```python
from build123d import *

# Parameters (mm, degrees)
F0_W      = 1348.74
F0_H      = 685.8
F1_DEPTH  = 25.4
F3_W      = 50.8
F3_H      = 317.5
F4_DEPTH  = 38.1
F5_W      = 50.8
F5_H      = 76.2
F6_DEPTH  = 660.4
F8_DEPTH  = 25.4
F9_W      = 1194.675028
F9_H      = 25.596991
F10_DEPTH = 304.8
F11_R     = 25.4
F12_R     = 25.4
F13_R     = 25.4
F14_R     = 25.4


with BuildPart() as f1:
    # F0 (on Top) → F1 (new body)
    with BuildSketch(Plane.XY):
        Rectangle(F0_W, F0_H)
    extrude(amount=F1_DEPTH)

    # F3 (on face) → F4 (join)
    with BuildSketch(Plane.XY.offset(25.4)):
        with Locations((-623.57, 44.45)):
            Rectangle(F3_W, F3_H)
        with Locations((623.57, 44.45)):
            Rectangle(F3_W, F3_H)
    extrude(amount=F4_DEPTH)

    # F5 (on face) → F6 (join)
    with BuildSketch(Plane.XY.offset(25.4)):
        with Locations((-623.57, -152.4)):
            Rectangle(F5_W, F5_H)
        with Locations((623.57, -152.4)):
            Rectangle(F5_W, F5_H)
    extrude(amount=F6_DEPTH)

    # F7 (on face) → F8 (join)
    with BuildSketch(Plane.XY.offset(685.8)):
        with BuildLine():
            ThreePointArc((-623.57, 241.3), (-641.530512, 233.860512), (-648.97, 215.9))
            Line((-648.97, 215.9), (-648.97, -241.3))
            ThreePointArc((-648.97, -241.3), (-641.530512, -259.260512), (-623.57, -266.7))
            ThreePointArc((-623.57, -266.7), (-605.609488, -259.260512), (-598.17, -241.3))
            Line((-598.17, -241.3), (-598.17, 215.9))
            ThreePointArc((-598.17, 215.9), (-605.609488, 233.860512), (-623.57, 241.3))
        make_face()
        with BuildLine():
            Line((648.97, -241.3), (648.97, 215.9))
            ThreePointArc((648.97, 215.9), (641.530512, 233.860512), (623.57, 241.3))
            ThreePointArc((623.57, 241.3), (605.609488, 233.860512), (598.17, 215.9))
            Line((598.17, 215.9), (598.17, -241.3))
            ThreePointArc((598.17, -241.3), (605.609488, -259.260512), (623.57, -266.7))
            ThreePointArc((623.57, -266.7), (641.530512, -259.260512), (648.97, -241.3))
        make_face()
    extrude(amount=F8_DEPTH)

    # F9 (on face) → F10 (join)
    with BuildSketch(Plane.XY.offset(25.4)):
        with Locations((-0.20507, -145.966001)):
            Rectangle(F9_W, F9_H)
    extrude(amount=F10_DEPTH)

    # F11
    f11_edges = [f1.edges().sort_by_distance(p)[0] for p in [
        (-674.37, 342.9, 12.7),
    ]]
    fillet(f11_edges, radius=F11_R)

    # F12
    f12_edges = [f1.edges().sort_by_distance(p)[0] for p in [
        (-674.37, -342.9, 12.7),
    ]]
    fillet(f12_edges, radius=F12_R)

    # F13
    f13_edges = [f1.edges().sort_by_distance(p)[0] for p in [
        (674.37, -342.9, 12.7),
    ]]
    fillet(f13_edges, radius=F13_R)

    # F14
    f14_edges = [f1.edges().sort_by_distance(p)[0] for p in [
        (674.37, 342.9, 12.7),
    ]]
    fillet(f14_edges, radius=F14_R)


solid = f1.part
```
The model under review builds one solid part; all positions refer to its coordinate system, in mm. A direction names the side the tool comes from. Round coordinates to 2 decimals unless told otherwise and drop trailing zeros. Order: outer loops, then holes, each group sorted by start corner. A loop starts at its lowest first (then second) coordinate and runs counter-clockwise, first axis right, second up.
(1) Take a section at A-A, the plane y = 17. State the section outline as (x, z) points.
Working result:
outline: (-674.37, 0) - (674.37, 0) - (674.37, 25.4) - (648.97, 25.4) - (648.97, 63.5) - (598.17, 63.5) - (598.17, 25.4) - (-598.17, 25.4) - (-598.17, 63.5) - (-648.97, 63.5) - (-648.97, 25.4) - (-674.37, 25.4) - close; (-648.97, 685.8) - (-598.17, 685.8) - (-598.17, 711.2) - (-648.97, 711.2) - close; (598.17, 685.8) - (648.97, 685.8) - (648.97, 711.2) - (598.17, 711.2) - close
(2) Wall thickness on L1, parallel to Z at x = -406, y = -289.5; L2, parallel to Y at x = 490.5, z = 177.5; L3, parallel to Y at x = 602.5, z = 188.5: over which ranges is each line inside the solid? List them lowest first.
Working result:
L1: z = 0 to 25.4
L2: y = -158.76 to -133.17
L3: y = -190.5 to -114.3
(3) Mouldability with a two-part tool opening along X and no side actions: class faces 5 (the face through (666.73, -335.66, 12.88)), 6 (the face through (598.17, -115, 341)), 7 (the face through (623, -9, 711.2)) as released by +X, released by -X, zero draft, split by the parting line, or undercut.
Working result:
face 5: released by +X
face 6: undercut
face 7: zero draft
(4) Tool access review of faces 1 (the face through (623, 47, 63.5)), 2 (the face through (-9, -133.168, 176)), 3 (the face through (623, -228, 685.8)), 4 (the face through (648.97, -115, 341)): name each direction out of +Z, -Z, +X, -X, +Y, -Y from which nothing blocks a thin tool from reaching the whole face with its end or side.
Working result:
face 1: +X, -X, +Y
face 2: +Z, +Y
face 3: +X, -X, -Y
face 4: +Z, +X, +Y, -Y
(5) Take a section at B-B, the plane z = 257. State the section outline as (x, y) points, plus the area to 3 significant figures.
Working result:
outline: (-648.97, -190.5) - (-598.17, -190.5) - (-598.17, -114.3) - (-648.97, -114.3) - close; (-597.54, -158.76) - (597.13, -158.76) - (597.13, -133.17) - (-597.54, -133.17) - close; (598.17, -190.5) - (648.97, -190.5) - (648.97, -114.3) - (598.17, -114.3) - close
area: 38,300 mm2
(6) Take a section at D-D, the plane x = 148.5. State the section outline as (y, z) points, plus the area to 3 significant figures.
Working result:
outline: (-342.9, 0) - (342.9, 0) - (342.9, 25.4) - (-133.17, 25.4) - (-133.17, 330.2) - (-158.76, 330.2) - (-158.76, 25.4) - (-342.9, 25.4) - close
area: 25,200 mm2
(7) For P1, Ø1.5, axis at x = 272, z = 323.5, coming from the +Y side; P2, Ø6, axis at y = -174, z = 157.5, coming from the +X side; P3, Ø1, axis at x = 147, y = 47, coming from the +Z side, all flat-tipped, find the tip position at first contact; note any pin that passes through.
Working result:
P1: stops at y = -133.17
P2: stops at x = 648.97
P3: stops at z = 25.4
(8) Take a section at C-C, the plane z = 605.5. State the section outline as (x, y) points, plus the area to 3 significant figures.
Working result:
outline: (-648.97, -190.5) - (-598.17, -190.5) - (-598.17, -114.3) - (-648.97, -114.3) - close; (598.17, -190.5) - (648.97, -190.5) - (648.97, -114.3) - (598.17, -114.3) - close
area: 7,740 mm2
